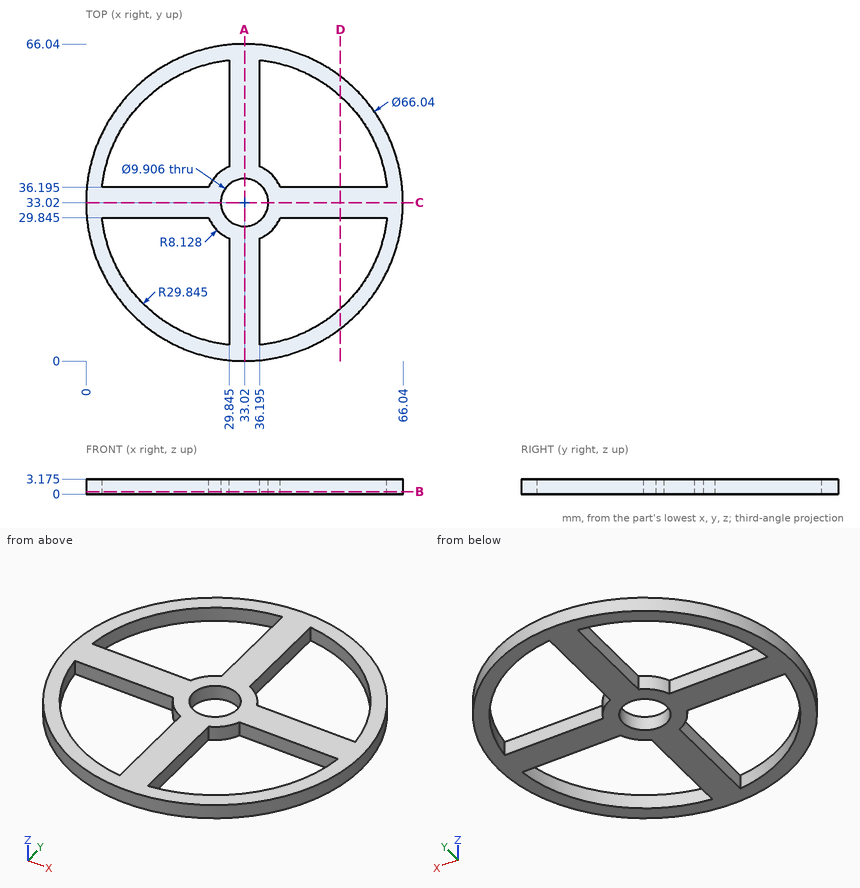
Design review of the part shown in the three views and the two pictorial views. Dimensions are in mm from the part's minimum x, y and z. Give positions to 0.01 mm unless a question says otherwise; leave off trailing zeros. Write each loop counter-clockwise with the first axis right and the second up, starting at its lowest first coordinate (ties: lowest second). Pieces come first, ordered by that corner, then holes.
Item 1: Take a section at D-D (x = 53). Give the boundary of the cut face in (y, z) (3 decimals), and give its area (3 significant figures).
Item 2: Insertion check: P1, Ø1.6, axis at y = 19, z = 2, coming from the -X side; P2, Ø1, axis at y = 46.5, z = 2, coming from the +X side; P3, Ø1.5, axis at y = 21.5, z = 2, coming from the -X side. Each pin has a flat end and moves straight along its axis. Give the tip position at first contact, or say it passes through.
Item 3: Take a section at A-A (x = 33.02). Give the boundary of the cut face in (y, z) (3 decimals), and give its area (3 significant figures).
Item 4: Take a section at B-B (z = 0.55). Give the boundary of the cut face in (x, y) (3 decimals), and give its area (3 significant figures).
Item 5: Wall thickness on probe 1 along Y at (x, z) = (33.02, 0.9); probe 2 along Y at (x, z) = (28, 0.3); probe 3 along X at (y, z) = (14, 1.6) (3 decimals): over which ranges is each line inside the solid? List them lowest first.
Established:
1. outline: (6.731, 0) - (10.85, 0) - (10.85, 3.175) - (6.731, 3.175) - close; (29.845, 0) - (36.195, 0) - (36.195, 3.175) - (29.845, 3.175) - close; (55.19, 0) - (59.309, 0) - (59.309, 3.175) - (55.19, 3.175) - close
1. area: 46.3 mm2
2. P1: stops at x = 2.76
2. P2: stops at x = 63.38
2. P3: stops at x = 1.81
3. outline: (0, 0) - (28.067, 0) - (28.067, 3.175) - (0, 3.175) - close; (37.973, 0) - (66.04, 0) - (66.04, 3.175) - (37.973, 3.175) - close
3. area: 178 mm2
4. outline: circle Ø66.04 at (33.02, 33.02); hole (3.344, 29.845) arc R29.845 ccw to (29.845, 3.344) - (29.845, 25.538) arc R8.128 cw to (25.538, 29.845) - close; hole (3.344, 36.195) - (25.538, 36.195) arc R8.128 cw to (29.845, 40.502) - (29.845, 62.696) arc R29.845 ccw to start; hole circle Ø9.906 at (33.02, 33.02); hole (36.195, 3.344) arc R29.845 ccw to (62.696, 29.845) - (40.502, 29.845) arc R8.128 cw to (36.195, 25.538) - close; hole (36.195, 40.502) arc R8.128 cw to (40.502, 36.195) - (62.696, 36.195) arc R29.845 ccw to (36.195, 62.696) - close
4. area: 1,310 mm2
5. probe 1: y = 0 to 28.07, 37.97 to 66.04
5. probe 2: y = 0.38 to 3.6, 26.63 to 39.41, 62.44 to 65.66
5. probe 3: x = 6.028 to 10.021, 29.845 to 36.195, 56.019 to 60.012
